Build history of the part. All positions in model axes, mm. A direction names the side the tool comes from. Give positions to 0.01 mm unless a question says otherwise; leave off trailing zeros. Loops run counter-clockwise (first coordinate to the right, second up) from the corner with the lowest first, then second, coordinate; pieces in that order, holes last. Notation, with made-up numbers: M -24,74 L 11,74 A18 ccw 11,93 Z; hole C -13.5,10 d4. An arc over 180 degrees is marked long. Put each result on its own line as item: value.
```python
from build123d import *

# Parameters (mm, degrees)
RUNROUTE_R           = 50.8
RUNEXTRUDE_DEPTH     = 95.25
OUTLETROUTE_R        = 50.8
OUTLETEXTRUDE_DEPTH  = 95.25
TEESHELL_START       = -95.25
TEESHELL_OUTLINE_R   = 45.0596
TEESHELL_DEPTH       = 190.5
TEESHELL_START_2     = -1e-07
TEESHELL_2_OUTLINE_R = 45.0596
TEESHELL_2_DEPTH     = 95.2500001
TEECHAMFER_SIZE      = 1.913466667


with BuildPart() as part:
    # RunRoute → RunExtrude (new body)
    with BuildSketch(Plane(origin=(0, 0, 0), x_dir=(0, 0, -1), z_dir=(1, 0, 0))):
        Circle(RUNROUTE_R)
    runextrude = extrude(amount=RUNEXTRUDE_DEPTH)

    # RunExtrudeMirror: RunExtrude across plane
    add(runextrude.mirror(Plane(origin=(0, 0, 0), x_dir=(0, 0, 1), z_dir=(1, 0, 0))))

    # OutletRoute → OutletExtrude (add)
    with BuildSketch(Plane(origin=(0, 0, 0), x_dir=(1, 0, 0), z_dir=(0, 1, 0))):
        with Locations(Location((0, 0, 0), (0, 0, 270))):
            Circle(OUTLETROUTE_R)
    extrude(amount=OUTLETEXTRUDE_DEPTH)

    # TeeShell: read off the stored shape, not the designer's step
    # TeeShell outline → TeeShell (cut)
    with BuildSketch(Plane.YZ.offset(TEESHELL_START)):
        Circle(TEESHELL_OUTLINE_R)
    extrude(amount=TEESHELL_DEPTH, mode=Mode.SUBTRACT)

    # TeeShell 2 outline → TeeShell 2 (cut)
    with BuildSketch(Plane(origin=(0, 0, 0), x_dir=(1, 0, 0), z_dir=(0, 1, 0)).offset(TEESHELL_START_2)):
        Circle(TEESHELL_2_OUTLINE_R)
    extrude(amount=TEESHELL_2_DEPTH, mode=Mode.SUBTRACT)

    # TeeChamfer
    # the kernel refuses this chamfer: 1.913466667 mm, written as the material it takes off along each edge
    with BuildSketch(Plane(origin=(95.25, 0, 0), x_dir=(0, 0, -1), z_dir=(0, -1, 0))) as teechamfer_piece_1:
        Polygon((50.8, -TEECHAMFER_SIZE), (50.8 - TEECHAMFER_SIZE, 0), (50.8, 0), align=None)
    revolve(axis=Axis((95.25, 0, 0), (1, 0, 0)), mode=Mode.SUBTRACT)
    with BuildSketch(Plane(origin=(-95.25, 0, 0), x_dir=(0, 0, -1), z_dir=(0, -1, 0))) as teechamfer_piece_2:
        Polygon((50.8, TEECHAMFER_SIZE), (50.8 - TEECHAMFER_SIZE, 0), (50.8, 0), align=None)
    revolve(axis=Axis((-95.25, 0, 0), (1, 0, 0)), mode=Mode.SUBTRACT)
    with BuildSketch(Plane(origin=(0, 95.25, 0), x_dir=(0, 0, 1), z_dir=(-1, 0, 0))) as teechamfer_piece_3:
        Polygon((50.8, -TEECHAMFER_SIZE), (50.8 - TEECHAMFER_SIZE, 0), (50.8, 0), align=None)
    revolve(axis=Axis((0, 95.25, 0), (0, 1, 0)), mode=Mode.SUBTRACT)


solid = part.part
```
Q1. Slice it at B-B (x = -55). List the corners of the cut face in (y, z).
Here are the results:
outline: C 0,0 d101.6; hole C 0,0 d90.12
Q2. Slice it at A-A (z = 0). List the corners of the cut face in (x, y), and give its area (3 significant figures).
Here are the results:
outline: M -95.25,-48.89 L -93.34,-50.8 L 93.34,-50.8 L 95.25,-48.89 L 95.25,-45.06 L -95.25,-45.06 Z; M -95.25,45.06 L -45.06,45.06 L -45.06,95.25 L -48.89,95.25 L -50.8,93.34 L -50.8,50.8 L -93.34,50.8 L -95.25,48.89 Z; M 45.06,45.06 L 95.25,45.06 L 95.25,48.89 L 93.34,50.8 L 50.8,50.8 L 50.8,93.34 L 48.89,95.25 L 45.06,95.25 Z
area: 2,170 mm²
Q3. Slice it at D-D (z = 27.5). State how many separate pieces and enclosed holes the cut face has, and give its area (3 significant figures).
Here are the results:
separate pieces: 3
enclosed holes: 0
area: 2,900 mm²
Q4. Probe line 1 (Z direction, x = 3.5, y = 0); line 2 (Y direction, x = -51, z = -25.5). List the from-to ranges inside material, lowest first. Write a range as from..to.
Here are the results:
line 1: -50.8..-45.06, 45.06..50.8
line 2: -43.94..-37.15, 37.15..43.94
Q5. Slice it at C-C (x = 0). List the corners of the cut face in (y, z).
Here are the results:
outline: M 0,-50.8 L 93.34,-50.8 L 95.25,-48.89 L 95.25,-45.06 L 0,-45.06 A45.06 cw 0,45.06 L 95.25,45.06 L 95.25,48.89 L 93.34,50.8 L 0,50.8 A50.8 ccw Z
Q6. Tool access for faces 1 (the cylindrical face through (1.307, -49.592, 11.012)), 2 (the flat face through (-43, 95.25, 14)): list every direction of +Z, -Z, +X, -X, +Y, -Y with a clear straight run to the whole face (end or side of a thin tool).
Here are the results:
face 1: none
face 2: +Z, -Z, +X, -X, +Y
Q7. Drop flat-ended pins along their axis: pin 1 Ø12 at (x, y) = (-41, -28) entering from +Z; pin 2 Ø3 at (x, y) = (-7.5, 25) entering from -Z; pin 3 Ø2 at (x, y) = (72, -6.5) entering from -Z; pin 4 Ø8 at (y, z) = (38.5, -11) entering from -X. Give the stop position or say it passes through.
Here are the results:
pin 1: z = 45.79
pin 2: z = -50.44
pin 3: z = -50.5
pin 4: through
Q8. Mould opens along Z. For faces 3 (the flat face through (95.25, -14, -43)), 4 (the cylindrical face through (-45.016, 57.542, -1.981)), 5 (the cylindrical face through (2.23, 56.39, -50.75)), 6 (the cylindrical face through (-1.334, -45.016, 1.981)) say: pulls with the +Z half, pulls with the -Z half, needs draft (parallel to the pull), parting line crosses it, or undercut.
Here are the results:
face 3: needs draft
face 4: undercut
face 5: parting line crosses it
face 6: undercut
